Work out the finished part from the listing and answer in its coordinate system (mm). Face numbers are marked on the shaded views. A direction names the side the tool comes from. Coordinates: 2 decimals unless noted, no trailing zeros. Write each loop counter-clockwise with the first axis right and the second up, starting at its lowest first coordinate (ties: lowest second). Pieces come first, ordered by that corner, then holes. Notation, with made-up numbers: (25.25, 75.5) - (72.25, 75.5) arc R16 ccw to (72.25, 92.5) - close; hole circle Ø6 at (-8.5, -19). An arc over 180 degrees is marked (long way). Use one line per item in the form item = value. Start each with the question number.
Item 1: Consider probe 1 along Z at (x, y) = (0, 214.5); probe 2 along Y at (x, z) = (6.5, 9); probe 3 along Z at (x, y) = (4.5, 201). Determine where each line is inside the solid, lowest interval first.
Item 2: A cutting plane is placed at C-C (y = 7). Write down the section's boundary in (x, z), then the cut area to 3 significant figures.
Item 3: A cutting plane is placed at D-D (z = 9). Write down the section's boundary in (x, y).
Item 4: Determine the mould class of the marked faces 3, 4 and 5 for opening direction Z: released by +Z, released by -Z, zero draft, split by the parting line, or undercut.
Item 5: A cutting plane is placed at A-A (x = 0). Write down the section's boundary in (y, z), then the cut area to 3 significant figures.
Item 6: For the marked faces 1 and 2, determine the directions among +Z, -Z, +X, -X, +Y, -Y from which every point of the face is accessible in a straight line to the end or side of a thin tool.
Item 7: A cutting plane is placed at B-B (z = 0). Write down the section's boundary in (x, y), then the cut area to 3 significant figures.
Item 8: Given pin 1 (6 mm diameter, centred on x = 3, z = -1.5, fed in from +Y); pin 2 (4 mm diameter, centred on y = 21.5, z = 6, fed in from -X); pin 3 (8 mm diameter, centred on y = 70.5, z = 5, fed in from +X); pin 4 (1.5 mm diameter, centred on x = 7, z = 9.5, fed in from -Y), each flat-ended and moving along its own axis, determine where each tip first touches the part or whether it passes through.
Autodesk Inventor part; units mm, degrees
ref_plane "YZ Plane" through (0, 0, 0) normal (1, 0, 0) x (0, 1, 0)
ref_plane "XZ Plane" through (0, 0, 0) normal (0, 1, 0) x (-1, 0, 0)
ref_plane "XY Plane" through (0, 0, 0) normal (0, 0, 1) x (1, 0, 0)
sketch "Skizze1" plane through (0, 0, 0) normal (0, 1, 0) x (-1, 0, 0)
  circle A0 centre (0, 0) radius 15
  dimension "d0" = 30
extrude "Extrusion1" add sketch "Skizze1" along normal blind 220
sketch "Skizze2" plane through (0, 0, 0) normal (0, -1, 0) x (1, 0, 0)
  circle A0 centre (0, 0) radius 6
  dimension "d3" = 12
extrude "Extrusion2" add sketch "Skizze2" along normal blind 24
thread "Gewinde1"
sketch "Skizze3" plane through (0, 220, 0) normal (0, 1, 0) x (1, 0, 0)
  circle A0 centre (0, 0) radius 15
hole "Bohrung1" at (0, 220, 0) direction (0, -1, 0) diameter 12 depth 20
properties part number "3" material "Kupfer, Legierung"
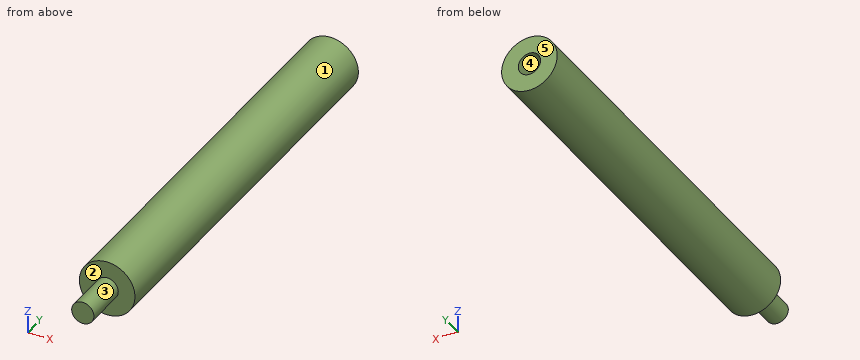
Answer:
q1.probe_1 = -15 to -6, 6 to 15
q1.probe_2 = 0 to 220
q1.probe_3 = -14.31 to -3.97, 3.97 to 14.31
q2.outline = circle Ø30 at (0, 0)
q2.area = 707 mm²
q3.outline = (-12, 0) - (12, 0) - (12, 220) - (-12, 220) - close
q4.face_3 = split by the parting line
q4.face_4 = undercut
q4.face_5 = zero draft
q5.outline = (-24, -6) - (0, -6) - (0, -15) - (220, -15) - (220, -6) - (200, -6) - (200, 6) - (220, 6) - (220, 15) - (0, 15) - (0, 6) - (-24, 6) - close
q5.area = 6,650 mm²
q6.face_1 = +Y, -Y
q6.face_2 = -Y
q7.outline = (-15, 0) - (-6, 0) - (-6, -24) - (6, -24) - (6, 0) - (15, 0) - (15, 220) - (6, 220) - (6, 200) - (-6, 200) - (-6, 220) - (-15, 220) - close
q7.area = 6,650 mm²
q8.pin_1 = 220
q8.pin_2 = -14.46
q8.pin_3 = 14.97
q8.pin_4 = 0
